Check sheet for the modelled part. Datum: model origin and axes. Units: mm. A direction names the side the tool comes from. Give positions to 0.01 mm unless a question says otherwise; leave off trailing zeros. Order: outer loops, then holes, each group sorted by start corner. A loop starts at its lowest first (then second) coordinate and runs counter-clockwise, first axis right, second up. Notation, with made-up numbers: (-3, -28.5) - (45, -28.5) arc R21 ccw to (45, -12.5) - close; hole circle Ø9 at (24.25, -3). An arc over 180 degrees is marked (long way). Answer in a Markdown table with one row per item.
Autodesk Inventor part; units mm, degrees
ref_plane "YZ Plane" through (0, 0, 0) normal (1, 0, 0) x (0, 1, 0)
ref_plane "XZ Plane" through (0, 0, 0) normal (0, 1, 0) x (-1, 0, 0)
ref_plane "XY Plane" through (0, 0, 0) normal (0, 0, 1) x (1, 0, 0)
sketch "Sketch1" plane through (0, 0, 0) normal (0, 0, 1) x (1, 0, 0)
  line L0 (0, 0) -> (20, 0)
  line L1 (20, 0) -> (20, 20)
  line L2 (20, 20) -> (0, 20)
  line L3 (0, 20) -> (0, 0)
  line L4 (-10, 5) -> (30, 5)
  line L5 (30, 5) -> (30, 15)
  line L6 (30, 15) -> (-10, 15)
  line L7 (-10, 15) -> (-10, 5)
  line L8 (-10, 5) -> (30, 15) construction
  line L9 (30, 5) -> (-10, 15) construction
  circle A0 centre (10, 10) radius 4.05
  point P0 (20, 5)
  point P1 (20, 15)
  dimension "d0" = 20
  dimension "d1" = 20
  dimension "d2" = 40
  dimension "d3" = 10
  dimension "d4" = 10
  dimension "d5" = 10
  dimension "d6" = 8.1
extrude "Extrusion1" add sketch "Sketch1" along normal blind 26 contours L3 L4 L1 L0 | L3 L6 L1 L4 | L1 L6 L5 L4 | L3 L2 L1 L6
chamfer "Chamfer1" distance 2 angle 45 6 edges at (20, 20, 13) (30, 15, 13) (30, 5, 13) (20, 0, 13) (0, 20, 13) (0, 0, 13)
fillet "Fillet1" radius 1 2 edges at (5.95, 10, 0) (5.95, 10, 26)
properties part number "Turret_Holder_2"
(1) Gauge pin test, flat ends, axial feed: P1, Ø3, axis at x = 25, y = 2.5, coming from the -Z side; P2, Ø0.9, axis at y = 16.5, z = 13.5, coming from the +X side; P3, Ø2.5, axis at x = 24.5, z = 6.5, coming from the -Y side; P4, Ø3.5, axis at y = 3.5, z = 9, coming from the +X side. Record the tip position at first contact, or that the pin passes through.
Geometry says:
| item | result |
|---|---|
| P1 | through |
| P2 | x = 20 |
| P3 | y = 5 |
| P4 | x = 28.25 |
(2) Cross-section at A-A, the plane y = 10. Record the cut outline in (x, z).
Geometry says:
| item | result |
|---|---|
| outline | (0, 0) - (4.95, 0) arc R1 ccw to (5.95, 1) - (5.95, 25) arc R1 ccw to (4.95, 26) - (0, 26) - close; (14.05, 1) arc R1 ccw to (15.05, 0) - (30, 0) - (30, 26) - (15.05, 26) arc R1 ccw to (14.05, 25) - close |
(3) Access from +Z, -Z, +X, -X, +Y, -Y to the whole of each face (thin tool, end or side, straight path). Record for faces 1 (the flat face through (20, 3, 13)), 2 (the flat face through (0, 10, 13)), 3 (the flat face through (24, 15, 13)).
Geometry says:
| item | result |
|---|---|
| face 1 | +Z, -Z, +X, -Y |
| face 2 | +Z, -Z, -X, +Y, -Y |
| face 3 | +Z, -Z, +X, +Y |
(4) Thickness scan on L1, parallel to Y at x = 10, z = 20; L2, parallel to X at y = 7.5, z = 20; L3, parallel to X at y = 13.25, z = 5.5. Record the ranges inside material, lowest first.
Geometry says:
| item | result |
|---|---|
| L1 | 0 to 5.95, 14.05 to 20 |
| L2 | 0 to 6.81, 13.19 to 30 |
| L3 | 0 to 7.58, 12.42 to 29.75 |
(5) Cross-section at C-C, the plane z = 23.25. Record the cut outline in (x, y), then the cut area to 3 significant figures.
Geometry says:
| item | result |
|---|---|
| outline | (0, 2) - (2, 0) - (18, 0) - (20, 2) - (20, 5) - (28, 5) - (30, 7) - (30, 13) - (28, 15) - (20, 15) - (20, 18) - (18, 20) - (2, 20) - (0, 18) - close; hole circle Ø8.1 at (10, 10) |
| area | 436 mm² |
(6) Mould release check, pull along X, two halves, no side actions. Record for faces 4 (the cylindrical face through (6.786, 12.464, 12.832)), 5 (the flat face through (29, 6, 13)), 6 (the flat face through (1, 19, 13)), 7 (the flat face through (15, 8, 26)): pulls with the +X half, pulls with the -X half, needs draft (parallel to the pull), parting line crosses it, or undercut.
Geometry says:
| item | result |
|---|---|
| face 4 | undercut |
| face 5 | pulls with the +X half |
| face 6 | pulls with the -X half |
| face 7 | needs draft |
(7) Cross-section at D-D, the plane y = 16.25. Record the cut outline in (x, z), then the cut area to 3 significant figures.
Geometry says:
| item | result |
|---|---|
| outline | (0, 0) - (20, 0) - (20, 26) - (0, 26) - close |
| area | 520 mm² |
(8) Cross-section at B-B, the plane x = 10. Record the cut outline in (y, z).
Geometry says:
| item | result |
|---|---|
| outline | (0, 0) - (4.95, 0) arc R1 ccw to (5.95, 1) - (5.95, 25) arc R1 ccw to (4.95, 26) - (0, 26) - close; (14.05, 1) arc R1 ccw to (15.05, 0) - (20, 0) - (20, 26) - (15.05, 26) arc R1 ccw to (14.05, 25) - close |
